Geometry check sheet. Reference: the model listing, model coordinates, mm. Face numbers are marked on the shaded views. A direction names the side the tool comes from. Round coordinates to 2 decimals unless told otherwise and drop trailing zeros. Order: outer loops, then holes, each group sorted by start corner. A loop starts at its lowest first (then second) coordinate and runs counter-clockwise, first axis right, second up. Notation, with made-up numbers: (82, 56.5) -> (119, 56.5) arc R23 cw to (119, 74.5) -> close; hole circle Ø1 at (73.25, 31). An arc over 180 degrees is marked (long way). Use a Markdown table: item, result. Add a question column.
Item 1: Material ranges on probe 1 along Y at (x, z) = (30, -6); probe 2 along Z at (x, y) = (34, 20); probe 3 along X at (y, z) = (7.75, -0.5), recorded low to high. Write a range as [from, to].
Item 2: Mould release check, pull along Y, two halves, no side actions. Record for the marked faces 4, 5 and 6: pulls with the +Y half, pulls with the -Y half, needs draft (parallel to the pull), parting line crosses it, or undercut.
Item 3: Sectioned sample at D-D, the plane z = -27. Record the cut outline in (x, y), and give its area (3 significant figures).
Item 4: Gauge pin test, flat ends, axial feed: pin 1 Ø4 at (x, z) = (-31, 1.5) entering from -Y; pin 2 Ø12 at (x, y) = (24, 7.5) entering from -Z; pin 3 Ø4 at (x, z) = (24, -1.5) entering from +Y. Record the tip position at first contact, or that the pin passes through.
Item 5: Sectioned sample at A-A, the plane x = 33. Record the cut outline in (y, z), and give its area (3 significant figures).
Item 6: Set-up check for the marked faces 1, 2 and 3: record each of +Z, -Z, +X, -X, +Y, -Y from which the full face is reachable in a straight line by a thin tool's end or side.
Item 7: Sectioned sample at B-B, the plane z = -5. Record the cut outline in (x, y), and give its area (3 significant figures).
Item 8: Sectioned sample at C-C, the plane y = 15.5. State how many separate pieces and enclosed holes the cut face has, and give its area (3 significant figures).
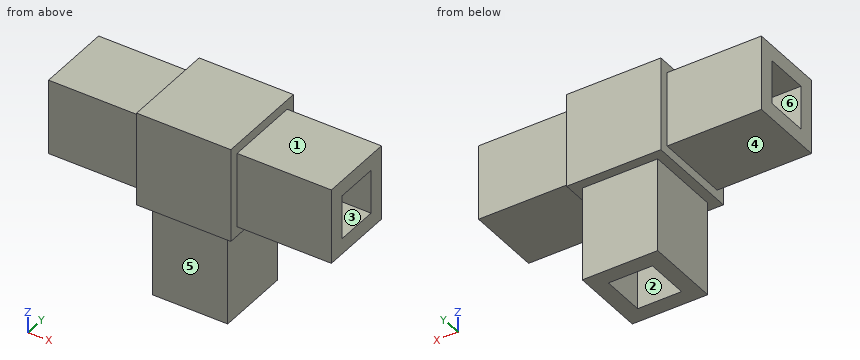
from build123d import *

# Parameters (mm, degrees)
CROQUIS1_W     = 30
CROQUIS1_H     = 30
EXTRUIR1_DEPTH = 30
CROQUIS2_W     = 30
CROQUIS2_H     = 30
CROQUIS2_W_2   = 24
CROQUIS2_H_2   = 24
EXTRUIR2_DEPTH = 30
CROQUIS3_W     = 30
CROQUIS3_H     = 30
CROQUIS3_W_2   = 24
CROQUIS3_H_2   = 24
EXTRUIR3_DEPTH = 30
CROQUIS5_W     = 30
CROQUIS5_H     = 30
CROQUIS5_W_2   = 24
CROQUIS5_H_2   = 24
EXTRUIR4_DEPTH = 30
VACIADO1_T     = -5


with BuildPart() as part:
    # Croquis1 → Extruir1 (new body)
    with BuildSketch(Plane(origin=(0, 0, 0), x_dir=(1, 0, 0), z_dir=(0, 1, 0))):
        with Locations((0, 30)):
            Rectangle(CROQUIS1_W, CROQUIS1_H)
        Rectangle(CROQUIS1_W, CROQUIS1_H)
        with Locations((30, 0)):
            Rectangle(CROQUIS1_W, CROQUIS1_H)
        with Locations((-30, 0)):
            Rectangle(CROQUIS1_W, CROQUIS1_H)
    extrude(amount=EXTRUIR1_DEPTH)

    # Croquis2 → Extruir2 (cut)
    with BuildSketch(Plane(origin=(45, 0, 0), x_dir=(0, 0, -1), z_dir=(1, 0, 0))):
        with Locations((0, 15)):
            Rectangle(CROQUIS2_W, CROQUIS2_H)
        with Locations((0, 15)):
            Rectangle(CROQUIS2_W_2, CROQUIS2_H_2, mode=Mode.SUBTRACT)
    extrude(amount=-EXTRUIR2_DEPTH, mode=Mode.SUBTRACT)

    # Croquis3 → Extruir3 (cut)
    with BuildSketch(Plane(origin=(0, 0, -45), x_dir=(-1, 0, 0), z_dir=(0, 0, -1))):
        with Locations((0, 15)):
            Rectangle(CROQUIS3_W, CROQUIS3_H)
        with Locations((0, 15)):
            Rectangle(CROQUIS3_W_2, CROQUIS3_H_2, mode=Mode.SUBTRACT)
    extrude(amount=-EXTRUIR3_DEPTH, mode=Mode.SUBTRACT)

    # Croquis5 → Extruir4 (cut)
    with BuildSketch(Plane.ZY.offset(45)):
        with Locations((0, 15)):
            Rectangle(CROQUIS5_W, CROQUIS5_H)
        with Locations((0, 15)):
            Rectangle(CROQUIS5_W_2, CROQUIS5_H_2, mode=Mode.SUBTRACT)
    extrude(amount=-EXTRUIR4_DEPTH, mode=Mode.SUBTRACT)

    # Vaciado1
    vaciado1_openings = [part.faces().sort_by_distance(p)[0] for p in [
        (45, 15, 0),
        (0, 15, -45),
        (-45, 15, 0),
    ]]
    offset(amount=VACIADO1_T, openings=vaciado1_openings, kind=Kind.INTERSECTION)


solid = part.part
Found:
| question | item | result |
|---|---|---|
| 1 | probe 1 | y = [3, 8], [22, 27] |
| 1 | probe 2 | z = [-12, -7], [7, 12] |
| 1 | probe 3 | x = [-45, -10], [10, 45] |
| 2 | face 4 | needs draft |
| 2 | face 5 | pulls with the -Y half |
| 2 | face 6 | undercut |
| 3 | outline | (-12, 3) -> (12, 3) -> (12, 27) -> (-12, 27) -> close; hole (-7, 8) -> (7, 8) -> (7, 22) -> (-7, 22) -> close |
| 3 | area | 380 mm2 |
| 4 | pin 1 | stops at y = 3 |
| 4 | pin 2 | stops at z = -12 |
| 4 | pin 3 | stops at y = 27 |
| 5 | outline | (3, -12) -> (27, -12) -> (27, 12) -> (3, 12) -> close; hole (8, -7) -> (22, -7) -> (22, 7) -> (8, 7) -> close |
| 5 | area | 380 mm2 |
| 6 | face 1 | +Z, +X, +Y, -Y |
| 6 | face 2 | -Z |
| 6 | face 3 | +X, -X |
| 7 | outline | (-45, 3) -> (-15, 3) -> (-15, 0) -> (15, 0) -> (15, 3) -> (45, 3) -> (45, 8) -> (10, 8) -> (10, 5) -> (-10, 5) -> (-10, 8) -> (-45, 8) -> close; (-45, 22) -> (-10, 22) -> (-10, 25) -> (10, 25) -> (10, 22) -> (45, 22) -> (45, 27) -> (15, 27) -> (15, 30) -> (-15, 30) -> (-15, 27) -> (-45, 27) -> close |
| 7 | area | 960 mm2 |
| 8 | separate pieces | 3 |
| 8 | enclosed holes | 0 |
| 8 | area | 1,190 mm2 |
